Autodesk Inventor part; units mm, degrees
ref_plane "pc_body_XY" through (7.5, 14, 0) normal (1, 0, 0) x (0, 0, -1)
ref_plane "pc_body_YZ" through (7.5, 14, 0) normal (0, 0, -1) x (0, 1, 0)
ref_plane "pc_body_ZX" through (7.5, 14, 0) normal (0, 1, 0) x (1, 0, 0)
sketch "Sketch_1" plane through (0, 0, 0) normal (1, 0, 0) x (0, 1, 0)
  line L0 (16.5, 46) -> (1, 46)
  arc A0 (1, 46) -> (0, 45) centre (1, 45) ccw
  line L1 (0, 45) -> (0, 43)
  line L2 (0, 43) -> (17.5, 43)
  line L3 (17.5, 43) -> (17.5, 30)
  line L4 (17.5, 30) -> (14, 30)
  line L5 (14, 30) -> (14, 20)
  line L6 (14, 20) -> (17.5, 20)
  line L7 (17.5, 20) -> (17.5, -20)
  line L8 (17.5, -20) -> (14, -20)
  line L9 (14, -20) -> (14, -30)
  line L10 (14, -30) -> (17.5, -30)
  line L11 (17.5, -30) -> (17.5, -43)
  line L12 (17.5, -43) -> (0, -43)
  line L13 (0, -43) -> (0, -45)
  arc A1 (0, -45) -> (1, -46) centre (1, -45) ccw
  line L14 (1, -46) -> (16.5, -46)
  arc A2 (16.5, -46) -> (19.5, -43) centre (16.5, -43) ccw
  line L15 (19.5, -43) -> (19.5, 43)
  arc A3 (19.5, 43) -> (16.5, 46) centre (16.5, 43) ccw
extrude "Extrusion1" add sketch "Sketch_1" along normal blind 1010
sketch "Sketch_3" plane through (7.5, 0, 0) normal (1, 0, 0) x (0, 0, -1)
  line L0 (-25, 21.1) -> (-25, 19.5)
  line L1 (-25, 19.5) -> (-30, 19.5)
  line L2 (-30, 19.5) -> (-30, 20.1)
  line L3 (-30, 20.1) -> (-27.4, 20.5)
  line L4 (-27.4, 20.5) -> (-27.4, 21.1)
  line L5 (-27.4, 21.1) -> (-25, 21.1)
  line L6 (-25, 21.1) -> (-25, 19.5)
revolve "Revolution1" add sketch "Sketch_3" angle 360 about axis through (7.5, 21.1, 25) along (0, 1, 0)
pattern_linear "Rectangular Pattern1" count 2 spacing 995 along (1, 0, 0) count 2 spacing 50 along (0, 0, -1) of "Revolution1"
ref_plane "pc_body_XY" through (7.5, 14, 0) normal (1, 0, 0) x (0, 0, -1)
ref_plane "pc_body_YZ" through (7.5, 14, 0) normal (0, 0, -1) x (0, 1, 0)
ref_plane "pc_body_ZX" through (7.5, 14, 0) normal (0, 1, 0) x (1, 0, 0)
properties part number "KR55-980-Protected Cover"
Could you check a few things on this model? Use its own coordinates, in mm. A direction names the side the tool comes from. Round coordinates to 2 decimals unless told otherwise and drop trailing zeros. Loops run counter-clockwise (first coordinate to the right, second up) from the corner with the lowest first, then second, coordinate; pieces in that order, holes last. Notation, with made-up numbers: M 15,27 L 21,27 A19 cw 21,44 Z; hole C -4,-1.75 d1. An arc over 180 degrees is marked long. Write item = value, one per line.
1. Thinking about a two-plate mould opening in Z: for faces 1 (the face through (498, 17.5, 0)), 2 (the face through (498, 9, 46)), 3 (the face through (0, 18, 0)), 4 (the face through (498, 9, -46)), which applies, +Z half, -Z half, draft (parallel to the pull), parting line (faces both ways), or undercut?
Results below:
face_1 = undercut
face_2 = +Z half
face_3 = draft
face_4 = -Z half
2. I want a section at A-A, the plane y = 6.75. Write out the boundary of the cut face in (x, z).
Results below:
outline = M 0,-46 L 1010,-46 L 1010,-43 L 0,-43 Z; M 0,43 L 1010,43 L 1010,46 L 0,46 Z
3. Which directions (+Z, -Z, +X, -X, +Y, -Y) give clear straight access to the entire face, cutting with the end or side of a thin tool? Please do faces 5 (the face through (498, 9, 43)), 6 (the face through (1010, 18, 0)).
Results below:
face_5 = +X, -X, -Y
face_6 = +Z, -Z, +X, +Y, -Y
4. I need wall thicknesses on probe 1 along Z at (x, y) = (495, 16.5); probe 2 along Z at (x, y) = (515, 2.25); probe 3 along Y at (x, z) = (867, 16). Which ranges of each line are inside material? Lowest first, please.
Results below:
probe_1 = -46 to -43, -30 to -20, 20 to 30, 43 to 46
probe_2 = -46 to -43, 43 to 46
probe_3 = 17.5 to 19.5
5. I want a section at C-C, the plane z = 11.5. Write out the boundary of the cut face in (x, y), and give its area (3 significant figures).
Results below:
outline = M 0,17.5 L 1010,17.5 L 1010,19.5 L 0,19.5 Z
area = 2,020 mm²
6. Will these pins go through, and if not, where does the flat tip stop? P1, Ø4, axis at x = 599, z = -34, coming from the -Y side; P2, Ø5, axis at x = 665, z = -13.5, coming from the +Y side; P3, Ø8, axis at x = 535.5, z = -26, coming from the -Y side.
Results below:
P1 = 17.5
P2 = 19.5
P3 = 14
7. I want a section at B-B, the plane x = 533.5. Write out the boundary of the cut face in (y, z).
Results below:
outline = M 0,-45 A1 ccw 1,-46 L 16.5,-46 A3 ccw 19.5,-43 L 19.5,43 A3 ccw 16.5,46 L 1,46 A1 ccw 0,45 L 0,43 L 17.5,43 L 17.5,30 L 14,30 L 14,20 L 17.5,20 L 17.5,-20 L 14,-20 L 14,-30 L 17.5,-30 L 17.5,-43 L 0,-43 Z
